Source: CAD feature listing. Evaluate the final solid. Frame: model axes, mm. Coordinates: 2 decimals unless noted, no trailing zeros. Write each loop counter-clockwise with the first axis right and the second up, starting at its lowest first coordinate (ties: lowest second). Pieces come first, ordered by that corner, then holes. Notation, with made-up numbers: (13.5, 85) - (46.5, 85) arc R30 cw to (46.5, 118) - close; hole circle Ø3 at (38, -15.5). An arc over 180 degrees is marked (long way). One line per question, with ' | ' between items. Start each with the question number.
Q1. Cut plane D-D, the plane x = -6. Return loops of the section in (y, z), plus the area to 3 significant figures.
Q2. Contact query for flat-ended pins moving along their axis: P1, Ø8, axis at x = -7, z = 23, coming from the -Y side; P2, Ø1.5, axis at x = -1, z = 25, coming from the +Y side; P3, Ø1.5, axis at y = -11, z = 11, coming from the -X side. Output: stop coordinate, or through.
Q3. Line query: line 1 (Z direction, x = -9.5, y = 3); line 2 (Z direction, x = 8.5, y = 10); line 3 (Y direction, x = 5, z = 18.25). Output: solid intervals per line, ascending.
Q4. Cut plane B-B, the plane z = 2.75. Return loops of the section in (x, y), plus the area to 3 significant figures.
Q5. Cut plane A-A, the plane x = 4.5. Return loops of the section in (y, z), plus the area to 3 significant figures.
Q6. Cut plane C-C, the plane y = 6.5. Return loops of the section in (x, z), plus the area to 3 significant figures.
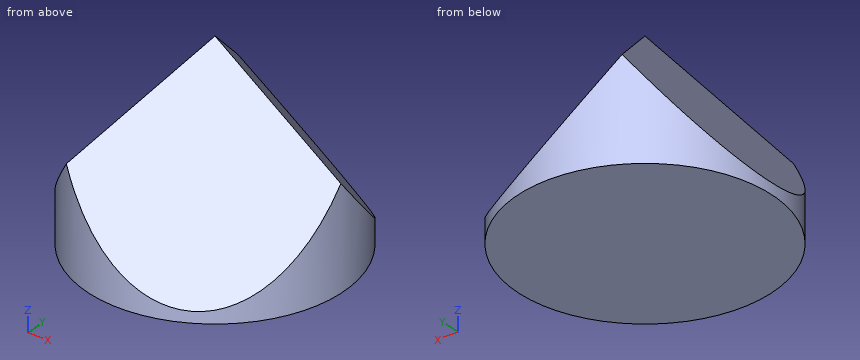
```python
from build123d import *

# Parameters (mm, degrees)
SKETCH_1_R          = 19
EXTRUDE_1_DEPTH     = 28.5
CUT_EXTRUDE_1_DEPTH = 24.5
CUT_EXTRUDE_2_DEPTH = 37
CUT_EXTRUDE_3_DEPTH = 28.5


with BuildPart() as part:
    # 草图1 → 凸台-拉伸1 (new body)
    with BuildSketch(Plane.XY):
        Circle(SKETCH_1_R)
    extrude(amount=EXTRUDE_1_DEPTH)

    # 草图2 → 切除-拉伸1 (cut, symmetric)
    with BuildSketch(Plane(origin=(0, 0, 0), x_dir=(1, 0, 0), z_dir=(0, 1, 0))):
        Polygon((0, -28.5), (-22.967769977, 3.974585824), (-22.967769977, -37.518896878), (0, -37.518896878), align=None)
    extrude(amount=CUT_EXTRUDE_1_DEPTH, both=True, mode=Mode.SUBTRACT)

    # 草图4 → 切除-拉伸2 (cut, symmetric)
    with BuildSketch(Plane(origin=(0, 0, 0), x_dir=(0.5, 0.866025404, 0), z_dir=(0.866025404, -0.5, 0))):
        Polygon((0, 28.5), (68.254426356, -68.006288105), (68.254426356, 39.794321241), (0, 39.794321241), align=None)
    extrude(amount=CUT_EXTRUDE_2_DEPTH, both=True, mode=Mode.SUBTRACT)

    # 草图5 → 切除-拉伸3 (cut, symmetric)
    with BuildSketch(Plane(origin=(0, 0, 0), x_dir=(0.5, -0.866025404, 0), z_dir=(-0.866025404, -0.5, 0))):
        Polygon((0, 28.5), (25.869335206, -8.07716649), (25.869335206, 34.9969783), (-0.936236718, 34.9969783), align=None)
    extrude(amount=CUT_EXTRUDE_3_DEPTH, both=True, mode=Mode.SUBTRACT)


solid = part.part
```
Reply:
1) outline: (-18.03, 0) - (18.03, 0) - (18.03, 10.67) - (10.39, 20.02) - (-10.39, 20.02) - (-18.03, 10.67) - close | area: 650 mm^2
2) P1: stops at y = -11.62 | P2: stops at y = 4.19 | P3: stops at x = -12.91
3) line 1: z = 0 to 15.07 | line 2: z = 0 to 10.25 | line 3: y = -5.48 to 5.48
4) outline: (-18.21, -5.42) arc R19 ccw to (4.42, -18.48) - (13.8, -13.06) arc R19 ccw to (13.8, 13.06) - (4.42, 18.48) arc R19 ccw to (-18.21, 5.42) - close | area: 1,120 mm^2
5) outline: (-18.46, 0) - (18.46, 0) - (18.46, 2.72) - (0, 25.32) - (-18.46, 2.72) - close | area: 517 mm^2
6) outline: (-17.85, 0) - (17.85, 0) - (17.85, 7.92) - (-3.75, 23.19) - (-17.85, 3.26) - close | area: 523 mm^2
